from build123d import *

# Parameters (mm, degrees)
SKETCH1_R               = 30
SKETCH1_R_2             = 2
SKETCH1_R_3             = 6
BOSS_EXTRUDE1_DEPTH     = 10
SKETCH2_R               = 2
CUT_EXTRUDE1_DEPTH      = 31
CUT_EXTRUDE1_DEPTH_BACK = 31
SKETCH3_R               = 5
CUT_EXTRUDE2_DEPTH      = 5


with BuildPart() as part:
    # Sketch1 → Boss-Extrude1 (new body)
    with BuildSketch(Plane(origin=(0, 0, 0), x_dir=(1, 0, 0), z_dir=(0, 1, 0))):
        Circle(SKETCH1_R)
        with Locations((20, 0)):
            Circle(SKETCH1_R_2, mode=Mode.SUBTRACT)
        with Locations((10, -17.320508076)):
            Circle(SKETCH1_R_2, mode=Mode.SUBTRACT)
        with Locations((-10, -17.320508076)):
            Circle(SKETCH1_R_2, mode=Mode.SUBTRACT)
        with Locations((-20, 0)):
            Circle(SKETCH1_R_2, mode=Mode.SUBTRACT)
        with Locations((-10, 17.320508076)):
            Circle(SKETCH1_R_2, mode=Mode.SUBTRACT)
        with Locations((10, 17.320508076)):
            Circle(SKETCH1_R_2, mode=Mode.SUBTRACT)
        Circle(SKETCH1_R_3, mode=Mode.SUBTRACT)
    extrude(amount=BOSS_EXTRUDE1_DEPTH)

    # Sketch2 → Cut-Extrude1 (cut, two sides)
    with BuildSketch(Plane.XY) as cut_extrude1_sk:
        with Locations((0, 5)):
            Circle(SKETCH2_R)
    extrude(amount=CUT_EXTRUDE1_DEPTH, mode=Mode.SUBTRACT)
    extrude(cut_extrude1_sk.sketch, amount=-CUT_EXTRUDE1_DEPTH_BACK, mode=Mode.SUBTRACT)

    # Sketch3 → Cut-Extrude2 (cut)
    with BuildSketch(Plane(origin=(0, 10, 0), x_dir=(1, 0, 0), z_dir=(0, 1, 0))):
        with Locations((-10, 17.320508076)):
            Circle(SKETCH3_R)
        with Locations((10, 17.320508076)):
            Circle(SKETCH3_R)
        with Locations((20, 0)):
            Circle(SKETCH3_R)
        with Locations((10, -17.320508076)):
            Circle(SKETCH3_R)
        with Locations((-10, -17.320508076)):
            Circle(SKETCH3_R)
        with Locations((-20, 0)):
            Circle(SKETCH3_R)
    extrude(amount=-CUT_EXTRUDE2_DEPTH, mode=Mode.SUBTRACT)


solid = part.part
Model file for the job. Use its own axes, mm. A direction names the side the tool comes from. Give positions to 0.01 mm unless a question says otherwise; leave off trailing zeros. Loops run counter-clockwise (first coordinate to the right, second up) from the corner with the lowest first, then second, coordinate; pieces in that order, holes last.
1) Saw through at D-D (x = 10.5). Write the cut outline in (y, z), plus the area to 3 significant figures.
2) Pull direction Y, two halves, no side cores. Call faces 1 (the flat face through (-0.4, 10, 6.2)), 2 (the cylindrical face through (12.688, 7.535, -21.537)), 3 (the cylindrical face through (0, 7, 18)), 4 (the flat face through (6.2, 0, -0.4)): +Y half, -Y half, draft (parallel to the pull), parting line (faces both ways), or undercut.
3) Wall check: line 1 (X direction, y = 1.55, z = 0); line 2 (Y direction, x = 0, z = -23); line 3 (X direction, y = 9.5, z = -13). Give the ranges that are in metal, low to high.
4) Saw through at A-A (x = 0). Write the cut outline in (y, z), plus the area to 3 significant figures.
5) Tool access for faces 5 (the cylindrical face through (9.566, 2.465, 19.273)), 6 (the cylindrical face through (-5.381, 7.535, 19.236)): list every direction of +Z, -Z, +X, -X, +Y, -Y with a clear straight run to the whole face (end or side of a thin tool).
6) Saw through at C-C (y = 8.5). Write the cut outline in (x, z).
7) Flat gauge pins, fed straight in: pin 1 Ø4.5 at (x, z) = (-20, 0) entering from +Y; pin 2 Ø2.5 at (x, z) = (20, 0) entering from +Y; pin 3 Ø3 at (x, y) = (16.5, 8) entering from -Z; pin 4 Ø2 at (x, y) = (6, 4.5) entering from +Z. Where does each tip first touch, or does it go through?
8) Saw through at B-B (z = 0). Write the cut outline in (x, y).
Answer block:
1. outline: (0, -28.1) - (10, -28.1) - (10, -22.3) - (5, -22.3) - (5, -19.26) - (0, -19.26) - close; (0, -15.38) - (5, -15.38) - (5, -12.35) - (10, -12.35) - (10, 12.35) - (5, 12.35) - (5, 15.38) - (0, 15.38) - close; (0, 19.26) - (5, 19.26) - (5, 22.3) - (10, 22.3) - (10, 28.1) - (0, 28.1) - close
1. area: 424 mm2
2. face 1: +Y half
2. face 2: draft
2. face 3: undercut
2. face 4: -Y half
3. line 1: x = -30 to -22, -18 to -6, 6 to 18, 22 to 30
3. line 2: y = 0 to 3, 7 to 10
3. line 3: x = -27.04 to -12.52, -7.48 to 7.48, 12.52 to 27.04
4. outline: (0, -30) - (3, -30) - (3, -6) - (0, -6) - close; (0, 6) - (3, 6) - (3, 30) - (0, 30) - close; (7, -30) - (10, -30) - (10, -6) - (7, -6) - close; (7, 6) - (10, 6) - (10, 30) - (7, 30) - close
4. area: 288 mm2
5. face 5: +Y, -Y
5. face 6: +Y
6. outline: circle Ø60 at (0, 0); hole circle Ø10 at (-20, 0); hole circle Ø10 at (-10, -17.32); hole circle Ø10 at (-10, 17.32); hole circle Ø12 at (0, 0); hole circle Ø10 at (10, -17.32); hole circle Ø10 at (10, 17.32); hole circle Ø10 at (20, 0)
7. pin 1: stops at y = 5
7. pin 2: passes through
7. pin 3: stops at z = -25.98
7. pin 4: stops at z = 29.58
8. outline: (-30, 0) - (-22, 0) - (-22, 5) - (-25, 5) - (-25, 10) - (-30, 10) - close; (-18, 0) - (-6, 0) - (-6, 10) - (-15, 10) - (-15, 5) - (-18, 5) - close; (6, 0) - (18, 0) - (18, 5) - (15, 5) - (15, 10) - (6, 10) - close; (22, 0) - (30, 0) - (30, 10) - (25, 10) - (25, 5) - (22, 5) - close
